Could you check a few things on this model? Use its own coordinates, in mm. A direction names the side the tool comes from. Coordinates: 2 decimals unless noted, no trailing zeros. Loops run counter-clockwise (first coordinate to the right, second up) from the corner with the lowest first, then second, coordinate; pieces in that order, holes last. Notation, with made-up numbers: M 15,59 L 22,59 A6 cw 22,66 Z; hole C 19.5,-24 d11. An arc over 180 degrees is marked long. Return JSON: item names as keys, results as strings. Group by question number.
from build123d import *

# Parameters (mm, degrees)
CYLINDER003_R          = 1
CYLINDER003_DEPTH      = 1
CYLINDER002_R          = 1
CYLINDER002_DEPTH      = 1
CYLINDER005_R          = 1
CYLINDER005_DEPTH      = 1
CYLINDER004_R          = 1
CYLINDER004_DEPTH      = 1
CUT002_PLACEMENT_ANGLE = 180
CYLINDER001_R          = 2.5
CYLINDER001_DEPTH      = 5
CYLINDER_R             = 3
CYLINDER_DEPTH         = 1


with BuildPart() as cilindro003:
    # Cylinder003 → Cylinder003 (new body)
    with BuildSketch(Plane(origin=(-7, 0, 0), x_dir=(1, 0, 0), z_dir=(0, 0, 1))):
        Circle(CYLINDER003_R)
    extrude(amount=CYLINDER003_DEPTH)


with BuildPart() as cut001:
    # Cylinder002 → Cylinder002 (new body)
    with BuildSketch(Plane(origin=(-8, 0, 0), x_dir=(1, 0, 0), z_dir=(0, 0, 1))):
        Circle(CYLINDER002_R)
    extrude(amount=CYLINDER002_DEPTH)

    # Cut001: cut Cilindro003
    add(cilindro003.part, mode=Mode.SUBTRACT)


with BuildPart() as cut001_1:
    # Cut001 placement: moved
    add(cut001.part.moved(Location((6, 3, 0))))


with BuildPart() as cilindro005:
    # Cylinder005 → Cylinder005 (new body)
    with BuildSketch(Plane(origin=(-7, 0, 0), x_dir=(1, 0, 0), z_dir=(0, 0, 1))):
        Circle(CYLINDER005_R)
    extrude(amount=CYLINDER005_DEPTH)


with BuildPart() as cut002:
    # Cylinder004 → Cylinder004 (new body)
    with BuildSketch(Plane(origin=(-8, 0, 0), x_dir=(1, 0, 0), z_dir=(0, 0, 1))):
        Circle(CYLINDER004_R)
    extrude(amount=CYLINDER004_DEPTH)

    # Cut002: cut Cilindro005
    add(cilindro005.part, mode=Mode.SUBTRACT)


with BuildPart() as cut002_1:
    # Cut002 placement: moved
    add(cut002.part.moved(Location((-6, 3, 0))).rotate(Axis((-6, 3, 0), (0, 0, 1)), CUT002_PLACEMENT_ANGLE))


with BuildPart() as cilindro001:
    # Cylinder001 → Cylinder001 (new body)
    with BuildSketch(Plane.XY.offset(-2)):
        Circle(CYLINDER001_R)
    extrude(amount=CYLINDER001_DEPTH)


with BuildPart() as fusion:
    # Cylinder → Cylinder (new body)
    with BuildSketch(Plane.XY):
        Circle(CYLINDER_R)
    extrude(amount=CYLINDER_DEPTH)

    # Cut: cut Cilindro001
    add(cilindro001.part, mode=Mode.SUBTRACT)

    # Fusion: union Cut001, Cut002
    add(cut001_1.part)
    add(cut002_1.part)


solid = fusion.part
(1) Imagine slicing it at C-C, the plane y = 2.75. Write out the boundary of the cut face in (x, z).
(2) Imagine slicing it at A-A, the plane x = 0. Write out the boundary of the cut face in (y, z), then the cut area to 3 significant figures.
(3) We'd pull the mould along X, two halves only. Please class faces 1 (the face through (1.98, 3.19, 0.49)), 2 (the face through (-0.9, 2.6, 0)): +X half, -X half, draft (parallel to the pull), parting line (faces both ways), or undercut.
(4) Will this pin go through, and if not, where does the flat tip stop? P1, Ø3, axis at x = -2, y = -1.5, coming from the -Z side.
(5) Imagine slicing it at D-D, the plane x = -2.35. Write out the boundary of the cut face in (y, z).
(6) For faces 3 (the face through (-1.977, 3.212, 0.493)), 4 (the face through (0.9, 2.6, 1)), which set-ups out of +Z, -Z, +X, -X, +Y, -Y let a thin tool reach every point of the face, with its end or its side?
(7) If I drill on L1, parallel to Y at x = 0, z = 0.35; L2, parallel to Y at x = -1.75, z = 0.1, over which ranges is the centre line in solid material (lowest first)? Write a range as [from, to].
Checks:
{
 "1": {"outline": "M -2.97,0 L -1.97,0 L -1.97,1 L -2.97,1 Z; M -1.2,0 L 1.2,0 L 1.2,1 L -1.2,1 Z; M 1.97,0 L 2.97,0 L 2.97,1 L 1.97,1 Z"},
 "2": {"outline": "M -3,0 L -2.5,0 L -2.5,1 L -3,1 Z; M 2.5,0 L 3,0 L 3,1 L 2.5,1 Z", "area": "1.00 mm²"},
 "3": {"face 1": "undercut", "face 2": "draft"},
 "4": {"P1": "z = 0"},
 "5": {"outline": "M -1.86,0 L -0.85,0 L -0.85,1 L -1.86,1 Z; M 0.85,0 L 1.86,0 L 1.86,1 L 0.85,1 Z; M 2.06,0 L 3.94,0 L 3.94,1 L 2.06,1 Z"},
 "6": {"face 3": "+Z, -Z", "face 4": "+Z, +X, -X, +Y, -Y"},
 "7": {"L1": "[-3, -2.5], [2.5, 3]", "L2": "[-2.44, -1.79], [1.79, 2.44], [3.66, 3.97]"}
}
